Drawing for the job (mm, zero at the part's lowest x, y, z). A direction names the side the tool comes from. Give positions to 0.01 mm unless a question says otherwise; leave off trailing zeros. Order: outer loops, then holes, each group sorted by start corner. A loop starts at its lowest first (then second) coordinate and runs counter-clockwise, first axis right, second up. Notation, with made-up numbers: (-5, 49) - (30, 49) arc R10 ccw to (30, 54) - close; hole circle Ø7 at (14.5, 23.25). An arc over 180 degrees is marked (long way). Use a Markdown table: item, result. Add a question column.
(1) Mould opens along Z. For the marked faces 1, 2 and 3 say: +Z half, -Z half, draft (parallel to the pull), parting line (faces both ways), or undercut.
(2) Slice it at D-D (x = 65). Write the cut outline in (y, z).
(3) Slice it at C-C (y = 8.5). Write the cut outline in (x, z), then the cut area to 3 significant figures.
(4) Slice it at B-B (x = 560). Write the cut outline in (y, z).
(5) Which spindle directions (+Z, -Z, +X, -X, +Y, -Y) get a long thin tool onto all of the face, cutting with end or side? Do the marked faces 4, 5, 6, 7 and 8. Say none if no direction does.
(6) Flat gauge pins, fed straight in: pin 1 (8 mm diameter, centred on x = 219, y = 85, fed in from +Z); pin 2 (20 mm diameter, centred on y = 39.5, z = 97, fed in from +X); pin 3 (5 mm diameter, centred on x = 122.5, y = 57, fed in from -Z). Where does each tip first touch, or does it go through?
(7) Slice it at A-A (y = 54). Write the cut outline in (x, z), then the cut area to 4 significant figures.
(8) Wall check: line 1 (Y direction, x = 560, z = 64); line 2 (Z direction, x = 516.5, y = 37); line 3 (Z direction, x = 320.5, y = 68). Give the ranges that are in metal, low to high.
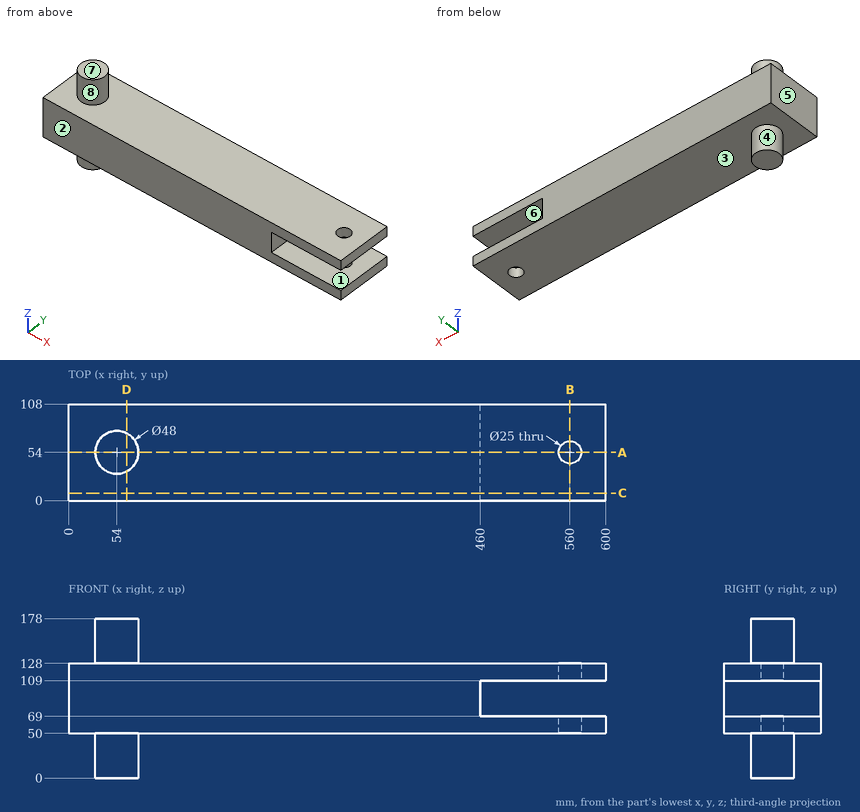
Solution:
| question | item | result |
|---|---|---|
| 1 | face 1 | undercut |
| 1 | face 2 | draft |
| 1 | face 3 | -Z half |
| 2 | outline | (0, 50) - (32.67, 50) - (32.67, 0) - (75.33, 0) - (75.33, 50) - (108, 50) - (108, 128) - (75.33, 128) - (75.33, 178) - (32.67, 178) - (32.67, 128) - (0, 128) - close |
| 3 | outline | (0, 50) - (600, 50) - (600, 69) - (460, 69) - (460, 109) - (600, 109) - (600, 128) - (0, 128) - close |
| 3 | area | 41,200 mm2 |
| 4 | outline | (0, 50) - (41.5, 50) - (41.5, 69) - (0, 69) - close; (0, 109) - (41.5, 109) - (41.5, 128) - (0, 128) - close; (66.5, 50) - (108, 50) - (108, 69) - (66.5, 69) - close; (66.5, 109) - (108, 109) - (108, 128) - (66.5, 128) - close |
| 5 | face 4 | -Z |
| 5 | face 5 | +Z, -Z, -X, +Y, -Y |
| 5 | face 6 | +X, +Y, -Y |
| 5 | face 7 | +Z, +X, -X, +Y, -Y |
| 5 | face 8 | +Z |
| 6 | pin 1 | z = 128 |
| 6 | pin 2 | x = 460 |
| 6 | pin 3 | z = 50 |
| 7 | outline | (0, 50) - (30, 50) - (30, 0) - (78, 0) - (78, 50) - (547.5, 50) - (547.5, 69) - (460, 69) - (460, 109) - (547.5, 109) - (547.5, 128) - (78, 128) - (78, 178) - (30, 178) - (30, 128) - (0, 128) - close; (572.5, 50) - (600, 50) - (600, 69) - (572.5, 69) - close; (572.5, 109) - (600, 109) - (600, 128) - (572.5, 128) - close |
| 7 | area | 45,050 mm2 |
| 8 | line 1 | 0 to 41.5, 66.5 to 108 |
| 8 | line 2 | 50 to 69, 109 to 128 |
| 8 | line 3 | 50 to 128 |
